Build history of the part. All positions in model axes, mm. A direction names the side the tool comes from. Round coordinates to 2 decimals unless told otherwise and drop trailing zeros. Order: outer loops, then holes, each group sorted by start corner. A loop starts at its lowest first (then second) coordinate and runs counter-clockwise, first axis right, second up. Notation, with made-up numbers: M -21.75,73.5 L 23.25,73.5 A32 ccw 23.25,99.5 Z; hole C -9.75,-8 d1. An arc over 180 degrees is marked long. Use CSV: the item, a comma, the result in double quotes.
from build123d import *

# Parameters (mm, degrees)
SKETCH_1_W               = 70
SKETCH_1_H               = 58
SKETCH_1_R               = 2.15
SKETCH_1_R_2             = 14
EXTRUDE_1_DEPTH          = 10
SKETCH_2_R               = 22
CUT_EXTRUDE_1_DEPTH      = 6
SKETCH_3_R               = 2.55
CUT_EXTRUDE_2_DEPTH      = 1
CUT_EXTRUDE_2_DEPTH_BACK = 59
SKETCH_4_R               = 2.05
CUT_EXTRUDE_3_DEPTH      = 1
CUT_EXTRUDE_3_DEPTH_BACK = 59
SKETCH_6_W               = 12.5
SKETCH_6_H               = 17.5
CUT_EXTRUDE_4_DEPTH      = 11
FILLET_1_R               = 1.5
SKETCH_7_W               = 3.5
SKETCH_7_H               = 10
CUT_EXTRUDE_5_DEPTH      = 1
CUT_EXTRUDE_5_DEPTH_BACK = 59
SKETCH_8_W               = 8.7
SKETCH_8_H               = 40
CUT_EXTRUDE_6_DEPTH      = 11
FILLET_3_R               = 1
SKETCH_9_W               = 43
SKETCH_9_H               = 6.5
CUT_EXTRUDE_7_DEPTH      = 11
FILLET_4_R               = 5
FILLET_5_R               = 2


with BuildPart() as part:
    # 草图1 → 凸台-拉伸1 (new body)
    with BuildSketch(Plane.XY):
        Rectangle(SKETCH_1_W, SKETCH_1_H)
        with Locations((17.5, 0)):
            Circle(SKETCH_1_R, mode=Mode.SUBTRACT)
        with Locations((0, -17.5)):
            Circle(SKETCH_1_R, mode=Mode.SUBTRACT)
        with Locations((-17.5, 0)):
            Circle(SKETCH_1_R, mode=Mode.SUBTRACT)
        with Locations((0, 17.5)):
            Circle(SKETCH_1_R, mode=Mode.SUBTRACT)
        Circle(SKETCH_1_R_2, mode=Mode.SUBTRACT)
    extrude(amount=EXTRUDE_1_DEPTH)

    # 草图2 → 切除-拉伸1 (cut)
    with BuildSketch(Plane.XY.offset(10)):
        Circle(SKETCH_2_R)
    extrude(amount=-CUT_EXTRUDE_1_DEPTH, mode=Mode.SUBTRACT)

    # 草图3 → 切除-拉伸2 (cut, two sides)
    with BuildSketch(Plane(origin=(0, 29, 0), x_dir=(1, 0, 0), z_dir=(0, 1, 0))) as cut_extrude_2_sk:
        with Locations((26.5, -5)):
            Circle(SKETCH_3_R)
    extrude(amount=CUT_EXTRUDE_2_DEPTH, mode=Mode.SUBTRACT)
    extrude(cut_extrude_2_sk.sketch, amount=-CUT_EXTRUDE_2_DEPTH_BACK, mode=Mode.SUBTRACT)

    # 草图4 → 切除-拉伸3 (cut, two sides)
    with BuildSketch(Plane(origin=(0, 29, 0), x_dir=(1, 0, 0), z_dir=(0, 1, 0))) as cut_extrude_3_sk:
        with Locations((-28.5, -5)):
            Circle(SKETCH_4_R)
    extrude(amount=CUT_EXTRUDE_3_DEPTH, mode=Mode.SUBTRACT)
    extrude(cut_extrude_3_sk.sketch, amount=-CUT_EXTRUDE_3_DEPTH_BACK, mode=Mode.SUBTRACT)

    # 草图6 → 切除-拉伸4 (cut, through all)
    with BuildSketch(Plane(origin=(0, 0, 0), x_dir=(-1, 0, 0), z_dir=(0, 0, -1))):
        with Locations((28.75, 20.25)):
            Rectangle(SKETCH_6_W, SKETCH_6_H)
        with Locations((28.75, -20.25)):
            Rectangle(SKETCH_6_W, SKETCH_6_H)
    extrude(amount=-CUT_EXTRUDE_4_DEPTH, mode=Mode.SUBTRACT)

    # 圆角1
    fillet_1_edges = [part.edges().sort_by_distance(p)[0] for p in [
        (-22.5, 11.5, 5),
        (-22.5, -11.5, 5),
    ]]
    fillet(fillet_1_edges, radius=FILLET_1_R)

    # 草图7 → 切除-拉伸5 (cut, two sides)
    with BuildSketch(Plane(origin=(0, 29, 0), x_dir=(1, 0, 0), z_dir=(0, 1, 0))) as cut_extrude_5_sk:
        with Locations((33.25, -5)):
            Rectangle(SKETCH_7_W, SKETCH_7_H)
    extrude(amount=CUT_EXTRUDE_5_DEPTH, mode=Mode.SUBTRACT)
    extrude(cut_extrude_5_sk.sketch, amount=-CUT_EXTRUDE_5_DEPTH_BACK, mode=Mode.SUBTRACT)

    # 草图8 → 切除-拉伸6 (cut, through all)
    with BuildSketch(Plane.XY.offset(10)):
        with Locations((27.15, 0)):
            Rectangle(SKETCH_8_W, SKETCH_8_H)
    extrude(amount=-CUT_EXTRUDE_6_DEPTH, mode=Mode.SUBTRACT)

    # 圆角3
    fillet_3_edges = [part.edges().sort_by_distance(p)[0] for p in [
        (22.8, 20, 5),
        (22.8, -20, 5),
    ]]
    fillet(fillet_3_edges, radius=FILLET_3_R)

    # 草图9 → 切除-拉伸7 (cut, through all)
    with BuildSketch(Plane.XY.offset(10)):
        with Locations((-1, -25.75)):
            Rectangle(SKETCH_9_W, SKETCH_9_H)
        with Locations((-1, 25.75)):
            Rectangle(SKETCH_9_W, SKETCH_9_H)
    extrude(amount=-CUT_EXTRUDE_7_DEPTH, mode=Mode.SUBTRACT)

    # 圆角4
    fillet_4_edges = [part.edges().sort_by_distance(p)[0] for p in [
        (-22.5, -22.5, 5),
        (-22.5, 22.5, 5),
    ]]
    fillet(fillet_4_edges, radius=FILLET_4_R)

    # 圆角5
    fillet_5_edges = [part.edges().sort_by_distance(p)[0] for p in [
        (20.5, -22.5, 5),
        (20.5, -29, 5),
        (20.5, 29, 5),
        (20.5, 22.5, 5),
    ]]
    fillet(fillet_5_edges, radius=FILLET_5_R)


solid = part.part
(1) Cut at D-D, the plane y = 16.5. Give the cut face in (x, z).
Answer block:
outline,"M -22.5,0 L -1.9,0 L -1.9,4 L -14.55,4 L -14.55,10 L -22.5,10 Z; M 1.9,0 L 22.8,0 L 22.8,10 L 14.55,10 L 14.55,4 L 1.9,4 Z"
(2) Wall check: line 1 (X direction, y = 0, z = 1.95); line 2 (Y direction, x = 0, z = 2.25); line 3 (Y direction, x = 0, z = 6.25). Give the ranges that are in metal, low to high. Write a range as from..to.
Answer block:
line 1,"x = -35..-19.65, -15.35..-14, 14..15.35, 19.65..22.8"
line 2,"y = -22.5..-19.65, -15.35..-14, 14..15.35, 19.65..22.5"
line 3,"y = -22.5..-22, 22..22.5"
(3) Drop flat-ended pins along their axis: pin 1 (5 mm diameter, centred on y = -18.5, z = 8, fed in from -X); pin 2 (3 mm diameter, centred on y = -9.5, z = 5, fed in from +X); pin 3 (4 mm diameter, centred on x = 17.5, y = 0, fed in from +Z); pin 4 (1.5 mm diameter, centred on x = -17, z = 7.5, fed in from +Y). Give the stop position or say it passes through.
Answer block:
pin 1,"stops at x = -22.5"
pin 2,"stops at x = 22.8"
pin 3,"passes through"
pin 4,"stops at y = 22.5"
(4) Cut at C-C, the plane x = -28.5. Give the cut face in (y, z), and give its area (3 significant figures).
Answer block:
outline,"M -11.5,0 L 11.5,0 L 11.5,2.95 L -11.5,2.95 Z; M -11.5,7.05 L 11.5,7.05 L 11.5,10 L -11.5,10 Z"
area,"136 mm²"
(5) Tool access for faces 1 (the face through (19.9, 23.07, 4.93)), 2 (the face through (-31, -11.5, 5)), 3 (the face through (29.3, 20, 5.1)): list every direction of +Z, -Z, +X, -X, +Y, -Y with a clear straight run to the whole face (end or side of a thin tool).
Answer block:
face 1,"+Z, -Z, -X, +Y"
face 2,"+Z, -Z, -X, -Y"
face 3,"+Z, -Z, +X"
(6) Cut at B-B, the plane x = 0. Give the cut face in (y, z).
Answer block:
outline,"M -22.5,0 L -19.65,0 L -19.65,4 L -22,4 L -22,10 L -22.5,10 Z; M -15.35,0 L -14,0 L -14,4 L -15.35,4 Z; M 14,0 L 15.35,0 L 15.35,4 L 14,4 Z; M 19.65,0 L 22.5,0 L 22.5,10 L 22,10 L 22,4 L 19.65,4 Z"
(7) Two-plate mould, pull along X, no slides. Class faces 4 (the face through (12.932, -5.362, 1.972)), 5 (the face through (0, 22.5, 5)), 6 (the face through (-10.1, 10.1, 4)), 7 (the face through (20.5, 26, 5)): released by +X, released by -X, zero draft, split by the parting line, or undercut.
Answer block:
face 4,"undercut"
face 5,"zero draft"
face 6,"undercut"
face 7,"released by -X"
(8) Cut at A-A, the plane y = 0. Give the cut face in (x, z), and give its area (3 significant figures).
Answer block:
outline,"M -35,0 L -19.65,0 L -19.65,4 L -22,4 L -22,10 L -35,10 Z; M -15.35,0 L -14,0 L -14,4 L -15.35,4 Z; M 14,0 L 15.35,0 L 15.35,4 L 14,4 Z; M 19.65,0 L 22.8,0 L 22.8,10 L 22,10 L 22,4 L 19.65,4 Z; hole C -28.5,5 d4.1"
area,"154 mm²"
